For this review, take the finished solid that the model builds, in its own axes (mm). A direction names the side the tool comes from. Give positions to 0.01 mm unless a question says otherwise; leave off trailing zeros. Write each loop counter-clockwise with the first axis right and the second up, starting at its lowest first coordinate (ties: lowest second). Pieces come first, ordered by that corner, then holes. Notation, with made-up numbers: (-8, -20.5) -> (19, -20.5) arc R32 ccw to (19, 18.5) -> close; hole circle Ø5 at (89.5, 84.25). An arc over 180 degrees is marked (long way). Write item = value, one per line.
```python
from build123d import *

# Parameters (mm, degrees)
F0_R          = 7.1
F1_DEPTH      = 60
F2_W          = 30
F2_H          = 32.2353386643
F3_DEPTH      = 25
F3_DEPTH_BACK = 25
F4_T          = -2.5


with BuildPart() as f1:
    # F0 (on Front) → F1 (new body)
    with BuildSketch(Plane.XZ):
        with BuildLine():
            Line((-55.5361600815, 234.910292219), (-55.535415078, -75.0897077801))
            ThreePointArc((-55.535415078, -75.0897077801), (-44.9776062474, -98.283221459), (-34.4179178598, -75.0905634563))
            Line((-34.4179178598, -75.0905634563), (-34.4186628633, 234.9094365428))
            Line((-34.4186628633, 234.9094365428), (-55.5361600815, 234.910292219))
        make_face()
        with Locations((-44.9770389706, -84.2832214705)):
            Circle(F0_R, mode=Mode.SUBTRACT)
    extrude(amount=F1_DEPTH)

    # F2 (on face) → F3 (cut, two sides)
    with BuildSketch(Plane(origin=(-55.535595536, 0, -0.0001334652), x_dir=(0, -1, 0), z_dir=(-1, 0, -2.4032e-06))) as f3_sk:
        with Locations((30, -88.0241336473)):
            Rectangle(F2_W, F2_H)
    extrude(amount=-F3_DEPTH, mode=Mode.SUBTRACT)
    extrude(f3_sk.sketch, amount=F3_DEPTH_BACK, mode=Mode.SUBTRACT)

    # F4
    f4_openings = [f1.faces().sort_by_distance(p)[0] for p in [
        (-44.977411, -30, 234.909864),
    ]]
    offset(amount=F4_T, openings=f4_openings, kind=Kind.INTERSECTION)


solid = f1.part
```
(1) Take a section at C-C (y = -8.5). Write out the cut boundary in (x, z).
Answers below:
outline = (-55.54, -75.09) arc R14 ccw (long way) to (-34.42, -75.09) -> (-34.42, 234.91) -> (-36.92, 234.91) -> (-36.92, -76.08) arc R11.5 cw (long way) to (-53.04, -76.08) -> (-53.04, 234.91) -> (-55.54, 234.91) -> close; circle Ø19.2 at (-44.98, -84.28); hole circle Ø14.2 at (-44.98, -84.28)
(2) Take a section at D-D (z = 2). Write out the cut boundary in (x, y).
Answers below:
outline = (-55.54, -60) -> (-34.42, -60) -> (-34.42, 0) -> (-55.54, 0) -> close; hole (-53.04, -57.5) -> (-36.92, -57.5) -> (-36.92, -2.5) -> (-53.04, -2.5) -> close
(3) Tool access review of faces 5 (the face through (-52.07, -52.4, -83.97)), 6 (the face through (-45, -47.5, -74)), 7 (the face through (-51.4, -15, -88.2)): name each direction out of +Z, -Z, +X, -X, +Y, -Y from which nothing blocks a thin tool from reaching the whole face with its end or side.
Answers below:
face_5 = +Y, -Y
face_6 = none
face_7 = -Z, +X, -X
(4) The part is to be moulded in two halves that separate along X. For faces 1 (the face through (-45, -57.5, 72)), 2 (the face through (-51.4, -45, -88.2)), 3 (the face through (-45.426, -52.395, -98.276)), 4 (the face through (-45.358, -52.43, -95.777)), say which applies: released by +X, released by -X, zero draft, split by the parting line, or undercut.
Answers below:
face_1 = undercut
face_2 = zero draft
face_3 = split by the parting line
face_4 = undercut
(5) Take a section at B-B (y = -36.5). Write out the cut boundary in (x, z).
Answers below:
outline = (-55.54, -71.91) -> (-34.42, -71.91) -> (-34.42, 234.91) -> (-36.92, 234.91) -> (-36.92, -69.41) -> (-53.04, -69.41) -> (-53.04, 234.91) -> (-55.54, 234.91) -> close
(6) For pin 1 (5 mm diameter, centred on y = -46, z = -23, fed in from -X); pin 2 (4 mm diameter, centred on y = -14, z = 112, fed in from +X), all flat-tipped, find the tip position at first contact; note any pin that passes through.
Answers below:
pin_1 = -55.54
pin_2 = -34.42
(7) To check wall thickness, follow probe 1 along X at (y, z) = (-38.5, 58.5); probe 2 along Z at (x, y) = (-53.25, -56); probe 3 along Y at (x, z) = (-48.5, 198). State the ranges of each line that lie inside material, in increasing order.
Answers below:
probe_1 = -55.54 to -53.04, -36.92 to -34.42
probe_2 = -95.58 to -92.27, -89.15 to -79.41, -76.3 to 234.91
probe_3 = -60 to -57.5, -2.5 to 0
(8) Take a section at A-A (x = -45). Count the separate pieces of the cut face and the enclosed holes in it, plus the area to 3 significant figures.
Answers below:
separate_pieces = 3
enclosed_holes = 2
area = 1,890 mm^2
